Source: CAD feature listing. Evaluate the final solid. Frame: model axes, mm. Face numbers are marked on the shaded views. Round coordinates to 2 decimals unless told otherwise and drop trailing zeros. Loops run counter-clockwise (first coordinate to the right, second up) from the corner with the lowest first, then second, coordinate; pieces in that order, holes last. Notation, with made-up numbers: M 58.25,22.25 L 91.25,22.25 A13 ccw 91.25,36.25 Z; hole C 1,6.5 d2. An arc over 180 degrees is marked long. One line per item, written item: value.
from build123d import *

# Parameters (mm, degrees)
BOSS_EXTRUDE1_DEPTH = 19.05
CUT_EXTRUDE1_DEPTH  = 7.62


with BuildPart() as part:
    # Sketch1 → Boss-Extrude1 (new body)
    with BuildSketch(Plane(origin=(0, 0, 0), x_dir=(1, 0, 0), z_dir=(0, 1, 0))):
        with BuildLine():
            Line((2.54, -0.381), (3.152057106, -0.381))
            ThreePointArc((3.152057106, -0.381), (0, -3.175), (-3.152057106, -0.381))
            Line((-3.152057106, -0.381), (-2.54, -0.381))
            Line((-2.54, -0.381), (-2.54, 0.381))
            Line((-2.54, 0.381), (-3.152057106, 0.381))
            ThreePointArc((-3.152057106, 0.381), (0, 3.175), (3.152057106, 0.381))
            Line((3.152057106, 0.381), (2.54, 0.381))
            Line((2.54, 0.381), (2.54, -0.381))
        make_face()
    extrude(amount=BOSS_EXTRUDE1_DEPTH)

    # Sketch2 → Cut-Extrude1 (cut)
    with BuildSketch(Plane(origin=(0, 19.05, 0), x_dir=(1, 0, 0), z_dir=(0, 1, 0))):
        with BuildLine():
            Line((-0.380189943, 0.928475362), (-0.380189943, 1.27))
            Line((-0.380189943, 1.27), (0.380189943, 1.27))
            Line((0.380189943, 1.27), (0.380189943, 0.928475362))
            ThreePointArc((0.380189943, 0.928475362), (1.0033, 0), (0.380189943, -0.928475362))
            Line((0.380189943, -0.928475362), (0.380189943, -1.27))
            Line((0.380189943, -1.27), (-0.380189943, -1.27))
            Line((-0.380189943, -1.27), (-0.380189943, -0.928475362))
            ThreePointArc((-0.380189943, -0.928475362), (-1.0033, 0), (-0.380189943, 0.928475362))
        make_face()
    extrude(amount=-CUT_EXTRUDE1_DEPTH, mode=Mode.SUBTRACT)


solid = part.part
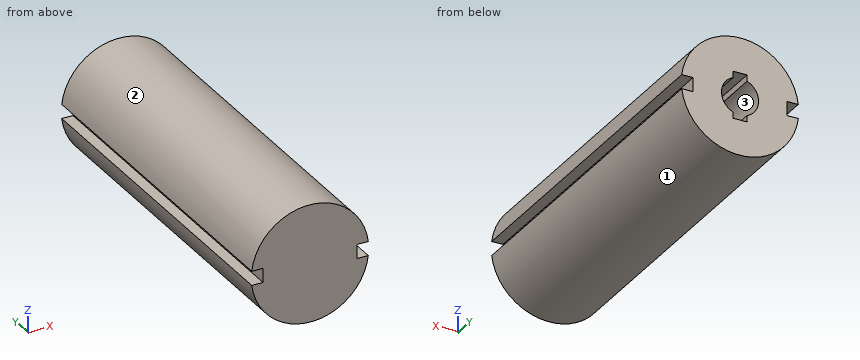
1. Section query B-B (y = 1.5). Return the cut outline in (x, z) (3 decimals).
Report:
outline: M -3.152,-0.381 A3.175 ccw 3.152,-0.381 L 2.54,-0.381 L 2.54,0.381 L 3.152,0.381 A3.175 ccw -3.152,0.381 L -2.54,0.381 L -2.54,-0.381 Z
2. Section query C-C (x = 0). Return the cut outline in (y, z) (3 decimals), and give its area (3 significant figures).
Report:
outline: M 0,-3.175 L 19.05,-3.175 L 19.05,-1.27 L 11.43,-1.27 L 11.43,1.27 L 19.05,1.27 L 19.05,3.175 L 0,3.175 Z
area: 102 mm2
3. Ray query, line 1 (X direction, y = 12, z = -0.75); line 2 (X direction, y = 4.5, z = 0); line 3 (Z direction, x = -0.5, y = 18). Return the intervals inside material, ascending. Write a range as [from, to].
Report:
line 1: x = [-3.09, -0.67], [0.67, 3.09]
line 2: x = [-2.54, 2.54]
line 3: z = [-3.14, -0.87], [0.87, 3.14]
4. Pull-direction query (Z, two-part tool) for the marked faces 1, 2 and 3; classes: released by +Z, released by -Z, zero draft, split by the parting line, or undercut.
Report:
face 1: released by -Z
face 2: released by +Z
face 3: undercut
5. Section query A-A (y = 11.75). Return the cut outline in (x, z) (3 decimals), and give its area (3 significant figures).
Report:
outline: M -3.152,-0.381 A3.175 ccw 3.152,-0.381 L 2.54,-0.381 L 2.54,0.381 L 3.152,0.381 A3.175 ccw -3.152,0.381 L -2.54,0.381 L -2.54,-0.381 Z; hole M -0.38,-1.27 L 0.38,-1.27 L 0.38,-0.928 A1.003 ccw 0.38,0.928 L 0.38,1.27 L -0.38,1.27 L -0.38,0.928 A1.003 ccw -0.38,-0.928 Z
area: 27.1 mm2
6. Section query D-D (z = -1.75). Return the cut outline in (x, y), and give its area (3 significant figures).
Report:
outline: M -2.65,0 L 2.65,0 L 2.65,19.05 L -2.65,19.05 Z
area: 101 mm2
7. Pin query (flat end, axial travel): pin 1 (1.5 mm diameter, centred on y = 7.5, z = 2.5, fed in from -X); pin 2 (0.7 mm diameter, centred on x = 3, y = 8, fed in from -Z). Return the tip coordinate at first contact, or that it passes through.
Report:
pin 1: stops at x = -2.65
pin 2: stops at z = -1.75
